Build history of the part. All positions in model axes, mm. Face numbers are marked on the shaded views. A direction names the side the tool comes from. Round coordinates to 2 decimals unless told otherwise and drop trailing zeros. Write each loop counter-clockwise with the first axis right and the second up, starting at its lowest first coordinate (ties: lowest second). Pieces come first, ordered by that corner, then holes. Notation, with made-up numbers: (33.5, 12.25) - (80.5, 12.25) arc R31 ccw to (80.5, 46.25) - close; hole circle Ø8 at (36.25, 44.5). An arc over 180 degrees is marked (long way). Answer as a JSON object with one key per item and string values. Group by question number.
Item 1: Slice it at C-C, the plane y = 22.25. List the corners of the cut face in (x, z).
Item 2: Flat gauge pins, fed straight in: pin 1 (2 mm diameter, centred on y = 22.5, z = 14, fed in from +X); pin 2 (3 mm diameter, centred on y = 58, z = 5.5, fed in from +X); pin 3 (2.5 mm diameter, centred on y = 30.85, z = 5.2, fed in from +X); pin 4 (2.5 mm diameter, centred on x = 29, z = 21.5, fed in from +Y). Where does each tip first touch, or does it go through?
Item 3: Slice it at B-B, the plane y = 11. List the corners of the cut face in (x, z), then the cut area to 3 significant figures.
Item 4: Slice it at A-A, the plane y = 30.85. List the corners of the cut face in (x, z).
Item 5: Slice it at D-D, the plane x = 34. Give the number of separate pieces and of enclosed holes in the cut face, then the cut area to 3 significant figures.
Item 6: Probe line 1 (Z direction, x = 38, y = 30); line 2 (X direction, y = 21.5, z = 20.25); line 3 (Y direction, x = 31.5, z = 23.5). List the from-to ranges inside material, lowest first. Write a range as from..to.
Item 7: Which spindle directions (+Z, -Z, +X, -X, +Y, -Y) get a long thin tool onto all of the face, cutting with end or side? Do the marked faces 1, 2, 3, 4 and 5. Say none if no direction does.
from build123d import *

# Parameters (mm, degrees)
SKETCH020_R             = 1.5
PAD012_DEPTH            = 18.8
SKETCH022_R             = 2.7
PAD010_DEPTH            = 8.7
SKETCH023_R             = 2.7
PAD011_DEPTH            = 9.3
PAD003_DEPTH            = 33
FILLET001_R             = 5
SKETCH021_R             = 2
PAD013_DEPTH            = 2
BODY005_PLACEMENT_ANGLE = 90


with BuildPart() as obj1:
    # Sketch020 → Pad012 (new body)
    with BuildSketch(Plane.XY):
        with BuildLine():
            Line((-8.25, -11.2), (8.25, -11.2))
            ThreePointArc((8.25, -11.2), (10.3713203436, -10.3213203436), (11.25, -8.2))
            Line((11.25, -8.2), (11.25, 25.8))
            Line((11.25, 25.8), (-11.25, 25.8))
            Line((-11.25, 25.8), (-11.25, -8.2))
            ThreePointArc((-11.25, -8.2), (-10.3713203436, -10.3213203436), (-8.25, -11.2))
        make_face()
        with Locations((-8.8, 19.85)):
            Circle(SKETCH020_R, mode=Mode.SUBTRACT)
        with Locations((8.8, 19.85)):
            Circle(SKETCH020_R, mode=Mode.SUBTRACT)
    extrude(amount=PAD012_DEPTH)

    # Sketch022 (on Face10 of Pad012) → Pad010 (join)
    with BuildSketch(Plane.XY.offset(18.8)):
        Circle(SKETCH022_R)
    extrude(amount=PAD010_DEPTH)

    # Sketch023 (on Face4 of Pad010) → Pad011 (join)
    with BuildSketch(Plane(origin=(0, 0, 0), x_dir=(1, 0, 0), z_dir=(0, 0, -1))):
        Circle(SKETCH023_R)
    extrude(amount=PAD011_DEPTH)

    # Sketch024 (on Face8 of Pad011) → Pad003 (join)
    with BuildSketch(Plane(origin=(0, 25.8, 0), x_dir=(-1, 0, 0), z_dir=(0, 1, 0))):
        with BuildLine():
            ThreePointArc((6.1808170981, 0), (11.25, 9.4), (6.1808170981, 18.8))
            Line((6.1808170981, 18.8), (-6.1808170981, 18.8))
            ThreePointArc((-6.1808170981, 18.8), (-11.25, 9.4), (-6.1808170981, 0))
            Line((6.1808170981, 0), (-6.1808170981, 0))
        make_face()
    extrude(amount=PAD003_DEPTH)

    # Fillet001
    fillet001_edges = [obj1.edges().sort_by_distance(p)[0] for p in [
        (-11.25, 58.8, 9.4),
        (0, 58.8, 18.8),
        (11.25, 58.8, 9.4),
        (0, 58.8, 0),
    ]]
    fillet(fillet001_edges, radius=FILLET001_R)

    # Sketch021 (on Face4 of Fillet001) → Pad013 (join)
    with BuildSketch(Plane(origin=(0, 0, 0), x_dir=(1, 0, 0), z_dir=(0, 0, -1))):
        with Locations((0, -11.25)):
            Circle(SKETCH021_R)
    extrude(amount=PAD013_DEPTH)


with BuildPart() as obj1_1:
    # Body005 placement: moved
    add(obj1.part.moved(Location((-45, 11, 14))).rotate(Axis((-45, 11, 14), (0, 1, 0)), BODY005_PLACEMENT_ANGLE))


with BuildPart() as part_mirroring:
    # Part__Mirroring: instance of obj1
    add(obj1_1.part.mirror(Plane(origin=(0, 34.7999992371, 13.9999961853), x_dir=(0, -1, 0), z_dir=(1, 0, -1.192e-07))))


solid = part_mirroring.part
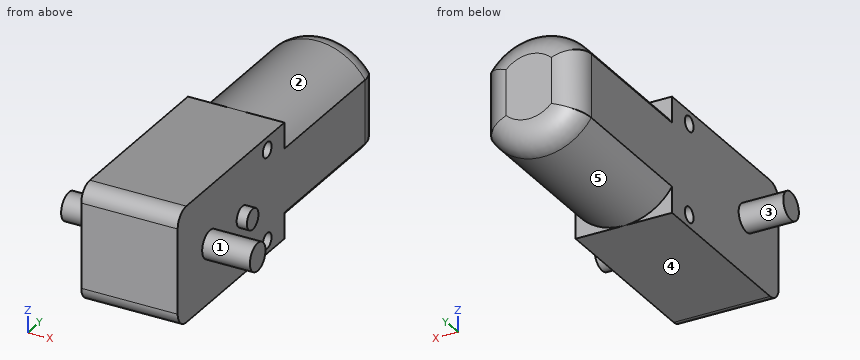
Geometry says:
{
 "1": {"outline": "(26.2, 2.75) - (45, 2.75) - (45, 12) - (47, 12) - (47, 16) - (45, 16) - (45, 25.25) - (26.2, 25.25) - close"},
 "2": {"pin 1": "stops at x = 47", "pin 2": "stops at x = 44.41", "pin 3": "passes through", "pin 4": "stops at y = 69.14"},
 "3": {"outline": "(17.5, 11.3) - (26.2, 11.3) - (26.2, 2.75) - (45, 2.75) - (45, 11.3) - (54.3, 11.3) - (54.3, 16.7) - (45, 16.7) - (45, 25.25) - (26.2, 25.25) - (26.2, 16.7) - (17.5, 16.7) - close", "area": "520 mm^2"},
 "4": {"outline": "(26.2, 2.75) - (45, 2.75) - (45, 3.7) - (26.2, 3.7) - close; (26.2, 6.7) - (45, 6.7) - (45, 21.3) - (26.2, 21.3) - close; (26.2, 24.3) - (45, 24.3) - (45, 25.25) - (26.2, 25.25) - close"},
 "5": {"separate pieces": "1", "enclosed holes": "2", "area": "1,540 mm^2"},
 "6": {"line 1": "z = 2.75..3.96, 6.44..21.56, 24.04..25.25", "line 2": "x = 26.2..45", "line 3": "y = 0.07..29.52, 32.18..67.67"},
 "7": {"face 1": "+X", "face 2": "+Z, +Y", "face 3": "-X", "face 4": "-Z, +X, -X, +Y, -Y", "face 5": "-Z, +Y"}
}
